Autodesk Inventor part; units mm, degrees
ref_plane "Work Plane1" through (20, 0, -31.25) normal (-1, 0, 0) x (0, 0, 1)
ref_plane "Work Plane2" through (44.948, 10, -2.6) normal (0, 0, -1) x (-1, 0, 0)
ref_plane "YZ Plane" through (0, 0, 0) normal (1, 0, 0) x (0, 1, 0)
sketch "Sketch1" plane through (0, 0, 0) normal (0, 1, 0) x (-1, 0, 0)
  line L0 (20, 31.25) -> (-20, 31.25)
  line L1 (-20, 31.25) -> (-20, -31.25)
  line L2 (-20, -31.25) -> (20, -31.25)
  line L3 (20, -31.25) -> (20, 31.25)
  line L4 (20, 31.25) -> (-20, -31.25) construction
  line L5 (-20, 31.25) -> (20, -31.25) construction
  point P0 (0, 0)
  dimension "d0" = 40
  dimension "d1" = 62.5
extrude "Extrusion1" add sketch "Sketch1" along normal blind 50
sketch "Sketch2" plane through (0, 50, 0) normal (0, 1, 0) x (1, 0, 0)
  line L0 (20, -31.25) -> (20, 31.25)
  line L1 (-20, -27.25) -> (20, -27.25)
  line L2 (20, -27.25) -> (20, 27.25)
  line L3 (20, 27.25) -> (-20, 27.25)
  line L4 (-20, 27.25) -> (-20, -27.25)
  line L5 (-20, -27.25) -> (20, 27.25) construction
  line L6 (20, -27.25) -> (-20, 27.25) construction
  line L7 (-20, -31.25) -> (20, -31.25)
  point P0 (0, 0)
  dimension "d4" = 4
extrude "Extrusion2" cut sketch "Sketch2" against normal blind 40
sketch "Sketch3" plane through (-20, 0, 31.25) normal (0, 0, 1) x (1, 0, 0)
  circle A0 centre (15, 31) radius 6.2
  line L0 (40, 10) -> (0, 10)
  line L1 (40, 10) -> (40, 50)
  line L2 (0, 0) -> (0, 50)
  point P0 (20, 0)
  point P1 (40, 30)
  dimension "d7" = 12.4
  dimension "d15" = 21
  dimension "d38" = 15
extrude "Extrusion3" cut sketch "Sketch3" against normal blind 8
sketch "Sketch4" plane through (20, 0, -31.25) normal (0, 0, -1) x (-1, 0, 0)
  circle A0 centre (25, 31) radius 6.2
  point P0 (20, 0)
extrude "Extrusion4" cut sketch "Sketch4" against normal blind 8
fillet "Fillet1" radius 2 2 edges at (0, 10, 27.25) (0, 10, -27.25)
sketch "Sketch5" plane through (20, 0, 31.25) normal (1, 0, 0) x (0, 0, -1)
  line L0 (4, 12) -> (4, 50)
  line L1 (0, 50) -> (4, 50)
  line L2 (0, 0) -> (0, 50)
  arc A0 (4, 12) -> (6, 10) centre (6, 12) ccw
  line L3 (0, 0) -> (62.5, 0)
  line L4 (56.5, 10) -> (6, 10)
  arc A1 (56.5, 10) -> (58.5, 12) centre (56.5, 12) ccw
  line L5 (58.5, 50) -> (58.5, 12)
  line L6 (62.5, 0) -> (62.5, 50)
  line L7 (58.5, 50) -> (62.5, 50)
  point P0 (31.25, 0)
extrude "Extrusion5" add sketch "Sketch5" along normal blind 30
sketch "Sketch6" plane through (0, 10, 0) normal (0, 1, 0) x (1, 0, 0)
  line L0 (9.748, 20.2) -> (44.948, 20.2)
  line L1 (44.948, 20.2) -> (44.948, -15)
  line L2 (44.948, -15) -> (9.748, -15)
  line L3 (9.748, -15) -> (9.748, 20.2)
  line L4 (9.748, 20.2) -> (44.948, -15) construction
  line L5 (44.948, 20.2) -> (9.748, -15) construction
  line L6 (-20, -25.25) -> (-20, 25.25)
  point P0 (0, 0)
  point P1 (27.348, 2.6)
  point P2 (-20, 0)
  point P3 (44.948, 2.6)
  dimension "d16" = 35.2
  dimension "d17" = 35.2
  dimension "d18" = 65
  dimension "d84" = 2.6
extrude "Extrusion6" cut sketch "Sketch6" against normal blind 3
sketch "Sketch10" plane through (0, 0, 0) normal (0, -1, 0) x (1, 0, 0)
  line L0 (44.948, 15) -> (9.748, 15)
  line L1 (44.948, -20.2) -> (44.948, 15)
  line L2 (9.748, -20.2) -> (44.948, -20.2)
  line L3 (9.748, 15) -> (9.748, -20.2)
  point P0 (0, 0)
  point P1 (27.348, -15.2)
  point P2 (27.348, -20.2)
  dimension "d37" = 5
hole "Hole1" at (27.348, 0, -15.2) direction (0, 1, 0) diameter 3.1 end through all countersink diameter 4 countersink angle 90
ref_plane "Work Plane1" through (20, 0, -31.25) normal (-1, 0, 0) x (0, 0, 1)
fillet "Fillet4" radius 2 4 edges at (-20, 50, -29.25) (50, 50, -29.25) (50, 50, 29.25) (-20, 50, 29.25)
sketch "Sketch16" plane through (50, 0, -31.25) normal (0, 0, -1) x (-1, 0, 0)
  line L0 (68, 50) -> (2, 50)
  arc A0 (2, 50) -> (0, 48) centre (2, 48) ccw
  line L1 (0, 0) -> (0, 48)
  line L2 (0, 12) -> (70, 12)
  line L3 (40, 50) -> (40, 12)
  point P0 (50, 0)
  dimension "d93" = 40
extrude "Extrusion14" cut sketch "Sketch16" against normal blind 4
fillet "Fillet5" radius 2 1 edges at (10, 50, -29.25)
sketch "Sketch17" plane through (-20, 0, 31.25) normal (0, 0, 1) x (1, 0, 0)
  line L0 (2, 50) -> (68, 50)
  line L1 (70, 48) -> (70, 0)
  arc A0 (70, 48) -> (68, 50) centre (68, 48) ccw
  line L2 (0, 12) -> (70, 12)
  line L3 (30, 50) -> (30, 12)
  point P0 (20, 0)
  dimension "d88" = 40
extrude "Extrusion15" cut sketch "Sketch17" against normal blind 4
fillet "Fillet6" radius 2 2 edges at (50, 12, 29.25) (50, 12, -29.25)
fillet "Fillet7" radius 2 1 edges at (10, 50, 29.25)
ref_plane "Work Plane2" through (44.948, 10, -2.6) normal (0, 0, -1) x (-1, 0, 0)
mirror "Mirror5" about plane through (44.948, 10, -2.6) normal (0, 0, -1) of "Hole1"
chamfer "Chamfer1" distance 6 angle 45 1 edges at (-20, 0, 0)
properties part number "base_engrane"
For this review, take the finished solid that the model builds, in its own axes (mm). A direction names the side the tool comes from. Round coordinates to 2 decimals unless told otherwise and drop trailing zeros. Write each loop counter-clockwise with the first axis right and the second up, starting at its lowest first coordinate (ties: lowest second). Pieces come first, ordered by that corner, then holes. Notation, with made-up numbers: M -19,89.25 L -4,89.25 A16 ccw -4,101.25 Z; hole C -36.5,4 d2. An arc over 180 degrees is marked long. One line per item, written item: value. Start each with the question number.
(1) Insertion check: pin 1 (4.5 mm diameter, centred on y = 31.5, z = -28.5, fed in from +X); pin 2 (4 mm diameter, centred on x = 27.348, z = 10, fed in from +Y); pin 3 (3 mm diameter, centred on x = 32, z = 29.5, fed in from +Y). Each pin has a flat end and moves straight along its axis. Give the tip position at first contact, or say it passes through.
(2) Wall thickness on line 1 (Y direction, x = -5, z = 28); line 2 (Z direction, x = 8.5, y = 32); line 3 (X direction, y = 7.5, z = 13): over which ranges is each line inside the solid? List them lowest first.
(3) We need section A-A (y = 23). Give the boundary of the cut face in (x, z), and give its area (3 significant figures).
(4) We need section D-D (y = 31). Give the boundary of the cut face in (x, z).
(5) Machinability: for faces 4 (the cylindrical face through (14.51, 10.6, -26.68)), 5 (the flat face through (27, 7, -3)), 6 (the flat face through (29, 12, 29)), which of the approach directions +Z, -Z, +X, -X, +Y, -Y give a long, thin tool a straight path to every point of the face, cutting with its end or side? Answer none if there is none.
(6) We need section C-C (x = -5). Give the boundary of the cut face in (y, z).
(7) We need section B-B (z = -15.2). Give the boundary of the cut face in (x, y).
(8) The part is to be moulded in two halves that separate along Z. For faces 1 (the flat face through (1.5, 30.7, 27.25)), 2 (the flat face through (7, 19, -31.25)), 3 (the cylindrical face through (-2.14, 25.5, 29.28)), say which applies: released by +Z, released by -Z, zero draft, split by the parting line, or undercut.
Result:
1. pin 1: x = 10
1. pin 2: y = 7
1. pin 3: y = 12
2. line 1: 0 to 24.8, 37.2 to 50
2. line 2: -31.25 to -27.25, 27.25 to 31.25
2. line 3: -20 to 9.75, 44.95 to 50
3. outline: M -20,-31.25 L 10,-31.25 L 10,-27.25 L -20,-27.25 Z; M -20,27.25 L 10,27.25 L 10,31.25 L -20,31.25 Z
3. area: 240 mm²
4. outline: M -20,-31.25 L -11.2,-31.25 L -11.2,-27.25 L -20,-27.25 Z; M -20,27.25 L -11.2,27.25 L -11.2,31.25 L -20,31.25 Z; M 1.2,-31.25 L 10,-31.25 L 10,-27.25 L 1.2,-27.25 Z; M 1.2,27.25 L 10,27.25 L 10,31.25 L 1.2,31.25 Z
5. face 4: +X, -X, +Y
5. face 5: +Y
5. face 6: +Z, -Z, +X, +Y
6. outline: M 0,-31.25 L 24.8,-31.25 L 24.8,-27.25 L 12,-27.25 A2 cw 10,-25.25 L 10,25.25 A2 cw 12,27.25 L 24.8,27.25 L 24.8,31.25 L 0,31.25 Z; M 37.2,-31.25 L 50,-31.25 L 50,-27.25 L 37.2,-27.25 Z; M 37.2,27.25 L 50,27.25 L 50,31.25 L 37.2,31.25 Z
7. outline: M -20,6 L -14,0 L 25.35,0 L 25.8,0.45 L 25.8,7 L 9.75,7 L 9.75,10 L -20,10 Z; M 28.9,0.45 L 29.35,0 L 50,0 L 50,10 L 44.95,10 L 44.95,7 L 28.9,7 Z
8. face 1: undercut
8. face 2: released by -Z
8. face 3: zero draft
